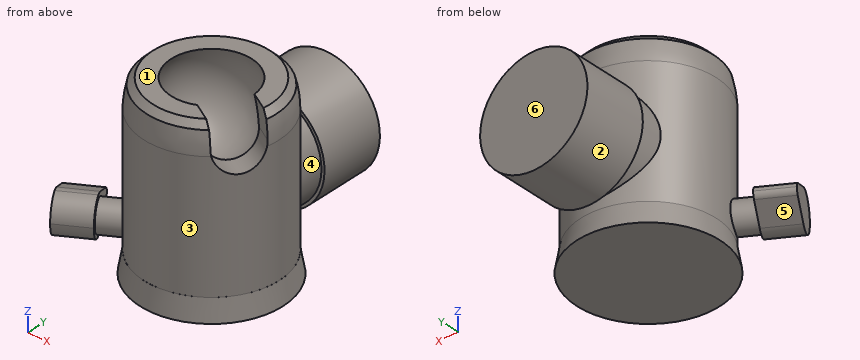
```python
from build123d import *
from OCP.BRepAlgoAPI import BRepAlgoAPI_Cut
from OCP.TopTools import TopTools_ListOfShape

# Parameters (mm, degrees)
SKETCH_1_R          = 23.25
EXTRUDE_1_DEPTH     = 7
EXTRUDE_1_TAPER     = 10
SKETCH_2_R          = 22
EXTRUDE_2_DEPTH     = 50.5
SKETCH_4_R          = 16.5
EXTRUDE_3_DEPTH     = 22.5
SKETCH_6_R          = 17.5
EXTRUDE_4_DEPTH     = 21
CUT_EXTRUDE_START   = -5.710511326
CUT_EXTRUDE_1_DEPTH = 12.710511326
SKETCH_10_R         = 4.8
EXTRUDE_5_DEPTH     = 12
EXTRUDE_6_DEPTH     = 11


with BuildPart() as part:
    # 草图1 → 凸台-拉伸1 (new body)
    with BuildSketch(Plane.XY):
        Circle(SKETCH_1_R)
    extrude(amount=EXTRUDE_1_DEPTH, taper=EXTRUDE_1_TAPER)

    # 草图2 → 凸台-拉伸2 (add)
    with BuildSketch(Plane.XY.offset(7)):
        Circle(SKETCH_2_R)
    extrude(amount=EXTRUDE_2_DEPTH)

    # 草图3 → 切除-旋转1 (revolve, cut)
    with BuildSketch(Plane(origin=(0, 0, 0), x_dir=(1, 0, 0), z_dir=(0, 1, 0))):
        with BuildLine():
            Line((21, -55.477297211), (22, -55.477297211))
            Line((22, -55.477297211), (22, -48.317565939))
            add(Edge.make_bspline(
                [(21, -55.477297211), (21.635397746, -53.150423877), (21.950433845, -50.732091094), (22, -48.317565939)],
                knots=[0, 0, 0, 0, 0.840917251, 0.840917251, 0.840917251, 0.840917251], degree=3))
        make_face()
        Polygon((19, -57.5), (22, -57.5), (22, -55.477297211), (21, -55.477297211), align=None)
    revolve(axis=Axis((0, 0, 57.5), (0, 0, -1)), mode=Mode.SUBTRACT)

    # 草图4 → 凸台-拉伸3 (add)
    with BuildSketch(Plane(origin=(0, 0, 0), x_dir=(1, 0, 0), z_dir=(0, 1, 0))):
        with Locations(Location((0, -26.5, 0), (0, 0, 90))):
            Circle(SKETCH_4_R)
    extrude(amount=EXTRUDE_3_DEPTH)

    # 草图6 → 凸台-拉伸4 (add)
    with BuildSketch(Plane(origin=(0, 22.5, 0), x_dir=(1, 0, 0), z_dir=(0, 1, 0))):
        with Locations(Location((0, -26.526637771, 0), (0, 0, 90))):
            Circle(SKETCH_6_R)
    extrude(amount=EXTRUDE_4_DEPTH)

    # 草图7 → 切除-旋转2 (revolve, cut)
    with BuildSketch(Plane(origin=(0, 0, 0), x_dir=(0, 0, -1), z_dir=(1, 0, 0))):
        with BuildLine():
            Line((-64.317565939, 0), (-32.317565939, 0))
            ThreePointArc((-32.317565939, 0), (-48.317565939, 16), (-64.317565939, 0))
        make_face()
    revolve(axis=Axis((0, 0, 57.5), (0, 0, -1)), mode=Mode.SUBTRACT)


with BuildPart() as cut_extrude_1_tool:
    # 切除-拉伸1: read off the stored shape, not the designer's step
    # 切除-拉伸1 outline → 切除-拉伸1 (new body)
    with BuildSketch(Plane(origin=(14.249995527, -8.227238754, -1.478e-06), x_dir=(0.49999999999999495, 0.8660254037844416, 0), z_dir=(0.8660254037844382, -0.49999999999999295, -8.981993465039313e-08)).offset(CUT_EXTRUDE_START)):
        with BuildLine():
            ThreePointArc((-7.5, 49.99999845), (3.87e-07, 42.5), (7.5, 49.999999225))
            Line((7.5, 49.999999225), (7.5, 57.5))
            Line((7.5, 57.5), (-7.5, 57.499999177))
            Line((-7.5, 57.499999177), (-7.5, 49.99999845))
        make_face()
    extrude(amount=CUT_EXTRUDE_1_DEPTH)


with BuildPart() as part_1:
    add(part.part)

    # 切除-拉伸1: cut by cut_extrude_1_tool, with a tolerance
    cut_extrude_1_stock = TopTools_ListOfShape()
    cut_extrude_1_stock.Append(part_1.part.wrapped)
    cut_extrude_1_tools = TopTools_ListOfShape()
    cut_extrude_1_tools.Append(cut_extrude_1_tool.part.wrapped)
    cut_extrude_1_cut = BRepAlgoAPI_Cut()
    cut_extrude_1_cut.SetArguments(cut_extrude_1_stock)
    cut_extrude_1_cut.SetTools(cut_extrude_1_tools)
    cut_extrude_1_cut.SetFuzzyValue(0.00001)
    cut_extrude_1_cut.Build()
    add(Compound.cast(cut_extrude_1_cut.Shape()).solids(), mode=Mode.REPLACE)

    # 草图10 → 凸台-拉伸5 (add)
    with BuildSketch(Plane(origin=(-14.25, -8.227241336, 0), x_dir=(0.500000000000007, -0.8660254037844346, 0), z_dir=(0.8660254037844346, 0.500000000000007, 0))):
        with Locations(Location((0, -13.6, 0), (0, 0, 180))):
            Circle(SKETCH_10_R)
    extrude(amount=-EXTRUDE_5_DEPTH)

    # 草图11 → 凸台-拉伸6 (add)
    with BuildSketch(Plane(origin=(-24.642304845, -14.227241336, 0), x_dir=(0, 0, 1), z_dir=(-0.8660254037844347, -0.500000000000007, 0))):
        with BuildLine():
            ThreePointArc((19.6, 0), (19.453472666, 1.31789899), (19.021047417, 2.571428571))
            ThreePointArc((19.021047417, 2.571428571), (16.807134903, 5.070925528), (13.6, 6))
            Line((13.6, 6), (13.6, 4.8))
            ThreePointArc((13.6, 4.8), (16.99411255, 3.39411255), (18.4, 0))
            ThreePointArc((18.4, 0), (16.99411255, -3.39411255), (13.6, -4.8))
            Line((13.6, -4.8), (13.6, -6))
            ThreePointArc((13.6, -6), (17.842640687, -4.242640687), (19.6, 0))
        make_face()
        with BuildLine():
            Line((13.6, 4.8), (13.6, 6))
            ThreePointArc((13.6, 6), (10.392865097, 5.070925528), (8.178952583, 2.571428571))
            ThreePointArc((8.178952583, 2.571428571), (8.529074472, -3.207134903), (13.6, -6))
            Line((13.6, -6), (13.6, -4.8))
            ThreePointArc((13.6, -4.8), (8.8, 0), (13.6, 4.8))
        make_face()
        with BuildLine():
            Line((19.021047417, 2.571428571), (15.407015806, 10.19047619))
            ThreePointArc((15.407015806, 10.19047619), (14.669044968, 11.023641843), (13.6, 11.333333333))
            Line((13.6, 11.333333333), (13.6, 6))
            ThreePointArc((13.6, 6), (16.807134903, 5.070925528), (19.021047417, 2.571428571))
        make_face()
        with BuildLine():
            Line((13.6, 6), (13.6, 11.333333333))
            ThreePointArc((13.6, 11.333333333), (12.530955032, 11.023641843), (11.792984194, 10.19047619))
            Line((11.792984194, 10.19047619), (8.178952583, 2.571428571))
            ThreePointArc((8.178952583, 2.571428571), (10.392865097, 5.070925528), (13.6, 6))
        make_face()
        with BuildLine():
            ThreePointArc((18.4, 0), (16.99411255, 3.39411255), (13.6, 4.8))
            Line((13.6, 4.8), (13.6, -4.8))
            ThreePointArc((13.6, -4.8), (16.99411255, -3.39411255), (18.4, 0))
        make_face()
        with BuildLine():
            Line((13.6, -4.8), (13.6, 4.8))
            ThreePointArc((13.6, 4.8), (8.8, 0), (13.6, -4.8))
        make_face()
    extrude(amount=EXTRUDE_6_DEPTH)


solid = part_1.part
```
The listing builds one solid part. Answer for the finished solid, in the listing's coordinates (mm). Face numbers are marked on the shaded views. A direction names the side the tool comes from. Round coordinates to 2 decimals unless told otherwise and drop trailing zeros. Order: outer loops, then holes, each group sorted by start corner. A loop starts at its lowest first (then second) coordinate and runs counter-clockwise, first axis right, second up. Notation, with made-up numbers: (23.5, 20) -> (50.5, 20) arc R13 cw to (50.5, 32) -> close; hole circle Ø4 at (13.5, 19). An arc over 180 degrees is marked (long way). Answer as CSV lines item,"result". Start each with the question number.
(1) The part is cut by section B-B (y = 30). Determine the outline of the cut face in (x, z), then the cut area to 3 significant figures.
(2) For a pull along Z with two mould halves and no side action, classify the marked faces 4, 5 and 6 as +Z half, -Z half, draft (parallel to the pull), parting line (faces both ways), or undercut.
(3) The part is cut by section A-A (z = 26.5). Determine the outline of the cut face in (x, y), then the cut area to 3 significant figures.
(4) A tool of negligible diameter and unlimited length cuts with its end or side. For the marked faces 1, 2 and 3, from which of +Z, -Z, +X, -X, +Y, -Y can it reach the whole face along a straight path? Write none if from no direction.
(5) Find the intervals of material crossed by probe 1 along X at (y, z) = (-9, 37); probe 2 along X at (y, z) = (-0.5, 16); probe 3 along X at (y, z) = (-2, 42), in increasing order. Write a range as from..to.
(6) The part is cut by section C-C (z = 6). Determine the outline of the cut face in (x, y), then the cut area to 3 significant figures.
(7) Flat-ended cylindrical pins translate along their axes: pin 1 Ø6 at (y, z) = (16.5, 35.5) entering from -X; pin 2 Ø10 at (y, z) = (-12, 6.5) entering from -X; pin 3 Ø10 at (x, y) = (12.5, 8) entering from -Z; pin 4 Ø1.5 at (y, z) = (33.5, 32) entering from +X. Find the tip coordinate at first contact, or state that the pin passes through.
Evaluation:
1,outline,"circle Ø35 at (0, 26.53)"
1,area,"962 mm²"
2,face 4,"undercut"
2,face 5,"-Z half"
2,face 6,"draft"
3,outline,"(-17.5, 22.5) -> (-16.5, 22.5) -> (-16.5, 14.55) arc R22 ccw (long way) to (16.5, 14.55) -> (16.5, 22.5) -> (17.5, 22.5) -> (17.5, 43.5) -> (-17.5, 43.5) -> close"
3,area,"2,350 mm²"
4,face 1,"+Z, +X, -X, +Y, -Y"
4,face 2,"+Y"
4,face 3,"none"
5,probe 1,"-20.07..-6.85, 6.85..20.07"
5,probe 2,"-21.99..21.99"
5,probe 3,"-21.91..-14.56, 14.56..21.91"
6,outline,"circle Ø44.38 at (0, 0)"
6,area,"1,550 mm²"
7,pin 1,"x = -17.37"
7,pin 2,"x = -38.93"
7,pin 3,"z = 0"
7,pin 4,"x = 16.85"
